Geometry: see drawing. Coordinates: mm, zero at the bounding-box minimum. A direction names the side the tool comes from. Round coordinates to 2 decimals unless told otherwise and drop trailing zeros. Loops run counter-clockwise (first coordinate to the right, second up) from the corner with the lowest first, then second, coordinate; pieces in that order, holes last. Notation, with made-up numbers: (23, 65) - (74, 65) arc R22 cw to (74, 91) - close; hole circle Ø5 at (-22, 23). An arc over 180 degrees is marked (long way). Write item = value, one per line. Start each with the question number.
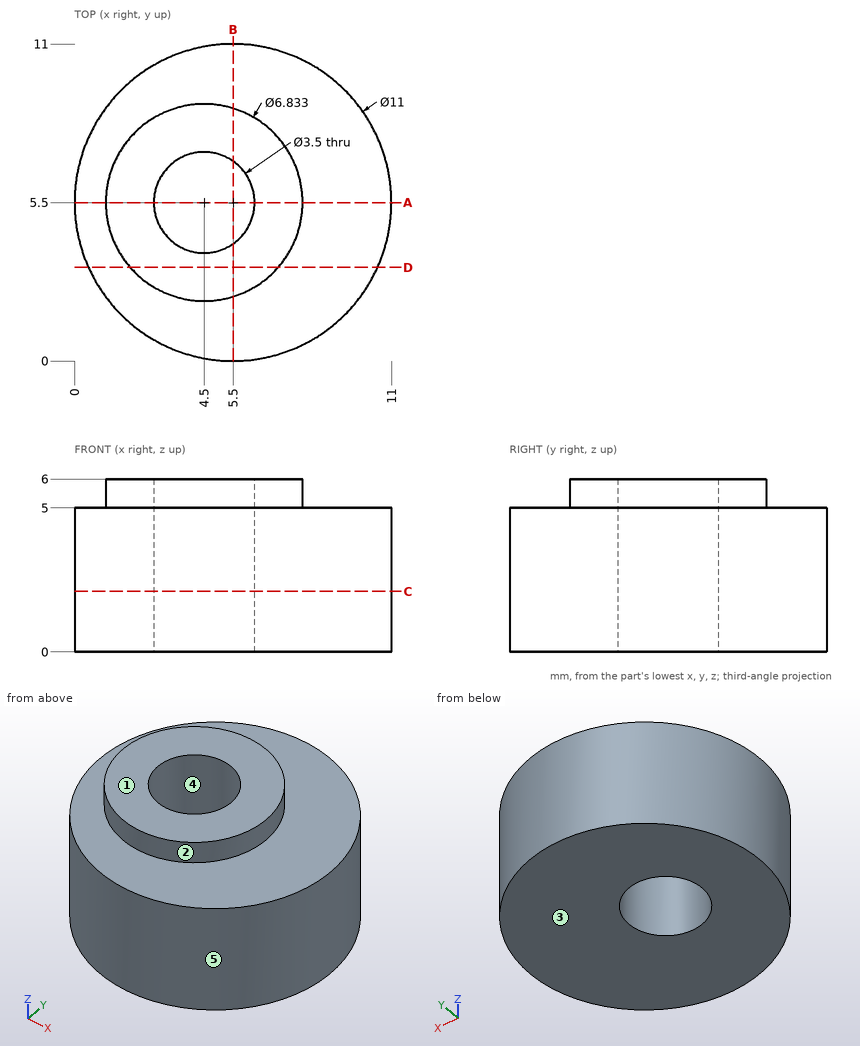
(1) Material intervals for line 1 along Z through (x, y) = (4.5, 1.5); line 2 along Y through (x, z) = (3, 3.5); line 3 along Y through (x, z) = (3.5, 5.6) (1 decimal), sorted ascending. Write a range as from..to.
(2) Access query for the marked faces 1 and 2. Directions: +Z, -Z, +X, -X, +Y, -Y. A direction counts if a zero-diameter tool reaches every point of the face in a straight line with its end or side. Return the directions, or none.
(3) Cut plane C-C (z = 2.1). Output: boundary loops of the cut face in (x, y), and give its area (3 significant figures).
(4) Mould query, pull axis X, two halves, no side actions, for the marked faces 3, 4 and 5. Classes: +X half, -X half, draft (parallel to the pull), parting line (faces both ways), or undercut.
(5) Cut plane A-A (y = 5.5). Output: boundary loops of the cut face in (x, z).
(6) Pin query (flat end, axial travel): P1, Ø2, axis at x = 5, y = 7, coming from the +Z side. Return the tip coordinate at first contact, or that it passes through.
(7) Cut plane D-D (y = 3.25). Output: boundary loops of the cut face in (x, z).
(8) Cut plane B-B (x = 5.5). Output: boundary loops of the cut face in (y, z), and give its area (3 significant figures).
Solution:
q1.line_1 = 0..5
q1.line_2 = 0.6..4.6, 6.4..10.4
q1.line_3 = 2.2..4.1, 6.9..8.8
q2.face_1 = +Z, +X, -X, +Y, -Y
q2.face_2 = +Z
q3.outline = circle Ø11 at (5.5, 5.5); hole circle Ø3.5 at (4.5, 5.5)
q3.area = 85.4 mm^2
q4.face_3 = draft
q4.face_4 = undercut
q4.face_5 = parting line
q5.outline = (0, 0) - (2.75, 0) - (2.75, 6) - (1.08, 6) - (1.08, 5) - (0, 5) - close; (6.25, 0) - (11, 0) - (11, 5) - (7.92, 5) - (7.92, 6) - (6.25, 6) - close
q6.P1 = 6
q7.outline = (0.48, 0) - (10.52, 0) - (10.52, 5) - (7.07, 5) - (7.07, 6) - (1.93, 6) - (1.93, 5) - (0.48, 5) - close
q8.outline = (0, 0) - (4.06, 0) - (4.06, 6) - (2.23, 6) - (2.23, 5) - (0, 5) - close; (6.94, 0) - (11, 0) - (11, 5) - (8.77, 5) - (8.77, 6) - (6.94, 6) - close
q8.area = 44.3 mm^2
